CAD build for the part. Positions are in the model's coordinates, mm. A direction names the side the tool comes from. Give positions to 0.01 mm unless a question says otherwise; leave off trailing zeros. Write each loop counter-clockwise with the first axis right and the second up, starting at its lowest first coordinate (ties: lowest second). Pieces come first, ordered by that corner, then holes. Notation, with made-up numbers: (2, 37) -> (25, 37) arc R6 cw to (25, 42) -> close; hole circle Ø9 at (8, 17). An arc over 180 degrees is marked (long way). Answer as a JSON object with one key per item and string values.
```python
from build123d import *

# Parameters (mm, degrees)
SKETCH_1_W                       = 137.5
SKETCH_1_H                       = 55
SM_BASE_FLANGE_1_DEPTH           = 1
SM_EDGE_FLANGE_3_STRIP_W         = 5.4732
SM_EDGE_FLANGE_3_STRIP_H         = 1
SM_EDGE_FLANGE_3_STRIP_CUT_DEPTH = 55
SM_EDGE_FLANGE_3_DEPTH           = 55
OTHER_START                      = -27.5
OTHER_1_DEPTH                    = 55
OTHER_1_2_DEPTH                  = 55


# Read off the part's stored shape, not the designer's step: Изгиб1
# Sheet-metal steps are written as plain solids
with BuildPart() as part:
    # Sketch 1 → Базовая кромка1 (new body)
    with BuildSketch(Plane.XY):
        with Locations((-68.75, 0)):
            Rectangle(SKETCH_1_W, SKETCH_1_H)
    extrude(amount=-SM_BASE_FLANGE_1_DEPTH)

    # Ребро-кромка3 strip (across the edge) → Ребро-кромка3 strip cut (cut)
    with BuildSketch(Plane(origin=(-137.5, 27.5, 0), x_dir=(1, 0, 0), z_dir=(0, -1, 0))):
        with Locations((-1, -0.5)):
            Rectangle(SM_EDGE_FLANGE_3_STRIP_W, SM_EDGE_FLANGE_3_STRIP_H)
    extrude(amount=SM_EDGE_FLANGE_3_STRIP_CUT_DEPTH, mode=Mode.SUBTRACT)

    # Ребро-кромка3 section (across the edge) → Ребро-кромка3 (add)
    with BuildSketch(Plane(origin=(-137.5, 27.5, 0), x_dir=(1, 0, 0), z_dir=(0, -1, 0))):
        with BuildLine():
            Line((0, 0.7366), (0, 69.7366))
            Line((0, 69.7366), (1, 69.7366))
            Line((1, 69.7366), (1, 0.7366))
            ThreePointArc((1, 0.7366), (1.215745145, 0.215745145), (1.7366, 0))
            Line((1.7366, 0), (1.7366, -1))
            ThreePointArc((1.7366, -1), (0.508638364, -0.491361636), (0, 0.7366))
        make_face()
    extrude(amount=SM_EDGE_FLANGE_3_DEPTH)

    # Other 1 outline → Other 1 (cut)
    with BuildSketch(Plane(origin=(0, 0, 0), x_dir=(1, 0, 0), z_dir=(0, 1, 0)).offset(OTHER_START)):
        with BuildLine():
            ThreePointArc((-136.5, -46.86049542), (-137.228828115, -46.219680493), (-137.5, -45.287854329))
            Line((-137.5, -45.287854329), (-137.5, -69.7366))
            Line((-137.5, -69.7366), (-136.5, -69.7366))
            Line((-136.5, -69.7366), (-136.5, -46.86049542))
        make_face()
    extrude(amount=OTHER_1_DEPTH, mode=Mode.SUBTRACT)

    # Other 1 2 outline → Other 1 2 (add)
    with BuildSketch(Plane(origin=(0, 0, 0), x_dir=(1, 0, 0), z_dir=(0, 1, 0)).offset(OTHER_START)):
        with BuildLine():
            Line((-136.5, -45.287854329), (-136.5, -46.86049542))
            ThreePointArc((-136.5, -46.86049542), (-136.140713558, -46.982969086), (-135.7634, -47.024454329))
            ThreePointArc((-135.7634, -47.024454329), (-135.242545145, -47.240199474), (-135.0268, -47.761054329))
            Line((-135.0268, -47.761054329), (-135.0268, -69.7366))
            Line((-135.0268, -69.7366), (-134.0268, -69.7366))
            Line((-134.0268, -69.7366), (-134.0268, -47.761054329))
            ThreePointArc((-134.0268, -47.761054329), (-134.535438364, -46.533092693), (-135.7634, -46.024454329))
            ThreePointArc((-135.7634, -46.024454329), (-136.284254855, -45.808709184), (-136.5, -45.287854329))
        make_face()
    extrude(amount=OTHER_1_2_DEPTH)

    # Зеркальное отражение1: part across plane


with BuildPart() as part_1:
    add(part.part)
    add(part.part.mirror(Plane(origin=(0, -27.5, -1), x_dir=(0, 0, 1), z_dir=(1, 0, 0))))


solid = part_1.part
```
1) Slice it at A-A (z = 21). List the corners of the cut face in (x, y), then the cut area to 3 significant figures.
Model answer:
{"outline": "(-137.5, -27.5) -> (-136.5, -27.5) -> (-136.5, 27.5) -> (-137.5, 27.5) -> close; (136.5, -27.5) -> (137.5, -27.5) -> (137.5, 27.5) -> (136.5, 27.5) -> close", "area": "110 mm2"}
2) Slice it at B-B (y = -20). List the corners of the cut face in (x, z).
Model answer:
{"outline": "(-137.5, 0.74) arc R1.74 ccw to (-135.76, -1) -> (135.76, -1) arc R1.74 ccw to (137.5, 0.74) -> (137.5, 45.29) arc R1.74 ccw to (135.76, 47.02) arc R0.74 cw to (135.03, 47.76) -> (135.03, 69.74) -> (134.03, 69.74) -> (134.03, 47.76) arc R1.74 ccw to (135.76, 46.02) arc R0.74 cw to (136.5, 45.29) -> (136.5, 0.74) arc R0.74 cw to (135.76, 0) -> (-135.76, 0) arc R0.74 cw to (-136.5, 0.74) -> (-136.5, 45.29) arc R0.74 cw to (-135.76, 46.02) arc R1.74 ccw to (-134.03, 47.76) -> (-134.03, 69.74) -> (-135.03, 69.74) -> (-135.03, 47.76) arc R0.74 cw to (-135.76, 47.02) arc R1.74 ccw to (-137.5, 45.29) -> close"}
3) Wall check: probe 1 along X at (y, z) = (-13, 59.5); probe 2 along X at (y, z) = (-2.5, 11.5); probe 3 along Z at (x, y) = (8.5, 0.5). Give the ranges that are in metal, low to high.
Model answer:
{"probe 1": "x = -135.03 to -134.03, 134.03 to 135.03", "probe 2": "x = -137.5 to -136.5, 136.5 to 137.5", "probe 3": "z = -1 to 0"}
4) Pin check, flat tips, straight feed: pin 1 (24 mm diameter, centred on y = 0.5, z = 60.5, fed in from -X); pin 2 (3 mm diameter, centred on x = 12.5, y = 18.5, fed in from +Z); pin 3 (17.5 mm diameter, centred on y = 8.5, z = 55.5, fed in from +X). Stop position of each tip, or through.
Model answer:
{"pin 1": "stops at x = -135.03", "pin 2": "stops at z = 0", "pin 3": "stops at x = 136.7"}
5) Slice it at C-C (x = -43). List the corners of the cut face in (y, z).
Model answer:
{"outline": "(-27.5, -1) -> (27.5, -1) -> (27.5, 0) -> (-27.5, 0) -> close"}
6) 3-axis set-ups, long thin cutter, end or side, ignore diameter. For faces 1 (the flat face through (-135.027, 0, 59)), 2 (the flat face through (-136.5, 0, 23)), 3 (the flat face through (135.027, 0, 59)): which of +Z, -Z, +X, -X, +Y, -Y reach the whole face in a straight line?
Model answer:
{"face 1": "+Z, -X, +Y, -Y", "face 2": "+Y, -Y", "face 3": "+Z, +X, +Y, -Y"}
7) Mould opens along Z. For faces 4 (the flat face through (136.5, 0, 23)), 5 (the flat face through (2, 0, -1)), 6 (the flat face through (-134.027, 0, 59)) say: released by +Z, released by -Z, zero draft, split by the parting line, or undercut.
Model answer:
{"face 4": "undercut", "face 5": "released by -Z", "face 6": "zero draft"}
